from build123d import *

# Parameters (mm, degrees)
CROQUIS1_R              = 150
CROQUIS1_R_2            = 125
SALIENTE_EXTRUIR1_DEPTH = 9
SALIENTE_EXTRUIR3_DEPTH = 9
CROQUIS3_R              = 1.5
SALIENTE_EXTRUIR4_DEPTH = 9


with BuildPart() as part:
    # Croquis1 → Saliente-Extruir1 (new body)
    with BuildSketch(Plane(origin=(0, 0, 0), x_dir=(1, 0, 0), z_dir=(0, 1, 0))):
        Circle(CROQUIS1_R)
        Circle(CROQUIS1_R_2, mode=Mode.SUBTRACT)
    extrude(amount=SALIENTE_EXTRUIR1_DEPTH)

    # Croquis2 → Saliente-Extruir3 (add)
    with BuildSketch(Plane(origin=(0, 0, 0), x_dir=(1, 0, 0), z_dir=(0, 1, 0))):
        Polygon((120.740728286, 32.352380638), (146.469530849, 32.352380638), (146.469530849, -32.352380638), (120.740728286, -32.352380638), (115.740728286, -31.012634676), (115.740728286, 31.012634676), align=None)
        Polygon((-88.388347648, -88.388347648), (-101.25274893, -110.670144277), (-45.216781919, -143.022524914), (-32.352380638, -120.740728286), (-31.012634676, -115.740728286), (-84.72809361, -84.72809361), align=None)
        Polygon((-32.352380638, 120.740728286), (-45.216781919, 143.022524914), (-101.25274893, 110.670144277), (-88.388347648, 88.388347648), (-84.72809361, 84.72809361), (-31.012634676, 115.740728286), align=None)
    extrude(amount=SALIENTE_EXTRUIR3_DEPTH)

    # Croquis3 → Saliente-Extruir4 (add)
    with BuildSketch(Plane(origin=(0, 0, 0), x_dir=(1, 0, 0), z_dir=(0, 1, 0))):
        Polygon((-70.549856067, 92.913902873), (-40, 40), (-40, -40), (-70.549856067, -92.913902873), (-40.549856067, -110.234410948), (0, -40), (40, -40), (40, -17.32), (115.740728286, -17.32), (115.740728286, 17.32), (40, 17.32), (40, 40), (0, 40), (-40.549856067, 110.234410948), align=None)
        with Locations((-35, 35)):
            Circle(CROQUIS3_R, mode=Mode.SUBTRACT)
        with Locations((35, 35)):
            Circle(CROQUIS3_R, mode=Mode.SUBTRACT)
        with Locations((35, -35)):
            Circle(CROQUIS3_R, mode=Mode.SUBTRACT)
        with Locations((-35, -35)):
            Circle(CROQUIS3_R, mode=Mode.SUBTRACT)
    extrude(amount=SALIENTE_EXTRUIR4_DEPTH)


solid = part.part
CAD build for the part. Positions are in the model's coordinates, mm. A direction names the side the tool comes from. Round coordinates to 2 decimals unless told otherwise and drop trailing zeros. Write each loop counter-clockwise with the first axis right and the second up, starting at its lowest first coordinate (ties: lowest second). Pieces come first, ordered by that corner, then holes. Notation, with made-up numbers: M -8,-11 L 47,-11 A19 ccw 47,20 Z; hole C 19.25,-8 d9. An arc over 180 degrees is marked long. Use a Markdown table: item, result. Add a question column.
1. Slice it at C-C on x = -58. Give the cut face in (y, z), then the cut area to 3 significant figures.
2. Drill centre lines: probe 1 along Z at (x, y) = (52, 8.5); probe 2 along Z at (x, y) = (-35, 4.25); probe 3 along X at (y, z) = (3.25, -65). Where is each one in solid material? Low to high.
3. Slice it at B-B on y = 5. Give the number of separate pieces and of enclosed holes in the cut face, then the cut area to 3 significant figures.
4. Flat gauge pins, fed straight in: P1, Ø2, axis at y = 3.5, z = 56.5, coming from the +X side; P2, Ø4, axis at x = 66, y = 6, coming from the -Z side; P3, Ø4, axis at y = 5.5, z = -114, coming from the -X side. Where does each tip first touch, or does it go through?
5. 3-axis set-ups, long thin cutter, end or side, ignore diameter. For faces 5 (the face through (78, 4, -17.32)), 6 (the face through (-2, 0, -2)): which of +Z, -Z, +X, -X, +Y, -Y reach the whole face in a straight line?
6. Pull direction Z, two halves, no side cores. Call faces 1 (the face through (20, 4, 40)), 2 (the face through (-19.527, 4.437, -148.724)), 3 (the face through (-2, 9, -2)), 4 (the face through (-55.061, 4.437, 66.087)): released by +Z, released by -Z, zero draft, split by the parting line, or undercut.
7. Slice it at A-A on z = 0. Give the cut face in (x, y), then the cut area to 4 significant figures.
Reply:
| question | item | result |
|---|---|---|
| 1 | outline | M 0,-138.33 L 9,-138.33 L 9,-71.18 L 0,-71.18 Z; M 0,71.18 L 9,71.18 L 9,138.33 L 0,138.33 Z |
| 1 | area | 1,210 mm^2 |
| 2 | probe 1 | z = -140.7 to -113.67, -17.32 to 17.32, 113.67 to 140.7 |
| 2 | probe 2 | z = -145.86 to -113.44, -100.62 to -36.5, -33.5 to 33.5, 36.5 to 100.62, 113.44 to 145.86 |
| 2 | probe 3 | x = -135.19 to -106.77, -54.43 to -14.43, 106.77 to 135.19 |
| 3 | separate pieces | 1 |
| 3 | enclosed holes | 7 |
| 3 | area | 37,000 mm^2 |
| 4 | P1 | stops at x = 139.35 |
| 4 | P2 | stops at z = -135.66 |
| 4 | P3 | stops at x = -99.78 |
| 5 | face 5 | +Y, -Y |
| 5 | face 6 | +Z, -Z, +X, -X, -Y |
| 6 | face 1 | undercut |
| 6 | face 2 | split by the parting line |
| 6 | face 3 | zero draft |
| 6 | face 4 | undercut |
| 7 | outline | M -150,0 L -125,0 L -125,9 L -150,9 Z; M -40,0 L 150,0 L 150,9 L -40,9 Z |
| 7 | area | 1,935 mm^2 |
